from build123d import *

# Parameters (mm, degrees)
F0_R     = 1.5875
F1_DEPTH = 1.524
F2_R     = 1.5875
F3_DEPTH = 4.7752


with BuildPart() as f1:
    # F0 (on Top) → F1 (new body)
    with BuildSketch(Plane.XY):
        with BuildLine():
            Line((-36.890476, -1.143), (-3.175, -2.38125))
            ThreePointArc((-3.175, -2.38125), (3.96875, 0), (-3.175, 2.38125))
            Line((-3.175, 2.38125), (-36.890476, 1.143))
            ThreePointArc((-36.890476, 1.143), (-43.0276, 0), (-36.890476, -1.143))
        make_face()
        with Locations((-39.8526, 0)):
            Circle(F0_R, mode=Mode.SUBTRACT)
        Circle(F0_R, mode=Mode.SUBTRACT)
    extrude(amount=F1_DEPTH)

    # F2 (on face) → F3 (join)
    with BuildSketch(Plane.XY.offset(1.524)):
        with Locations((-39.8526, 0)):
            Circle(F2_R)
        Circle(F2_R)
    extrude(amount=-F3_DEPTH)


solid = f1.part
Part model, mm, in its own coordinate system. A direction names the side the tool comes from. Coordinates: 2 decimals unless noted, no trailing zeros. Write each loop counter-clockwise with the first axis right and the second up, starting at its lowest first coordinate (ties: lowest second). Pieces come first, ordered by that corner, then holes. Notation, with made-up numbers: M 69.25,24 L 96.25,24 A16 cw 96.25,53 Z; hole C 75.5,83 d5. An arc over 180 degrees is marked long. Return JSON: item names as keys, results as strings.
1. Flat gauge pins, fed straight in: pin 1 Ø3 at (x, y) = (-20, 2.5) entering from -Z; pin 2 Ø1 at (x, z) = (-28.5, 0) entering from +Y. Where does each tip first touch, or does it go through?
Determined:
{"pin 1": "z = 0", "pin 2": "y = 1.47"}
2. Saw through at C-C, the plane z = -0.5. Write the cut outline in (x, y) (1 decimal).
Determined:
{"outline": "C -39.9,0 d3.2; C 0,0 d3.2"}
3. 3-axis set-ups, long thin cutter, end or side, ignore diameter. For faces 3 (the face through (-20.269, -1.753, 0.751)), 4 (the face through (-0.34, -1.55, -1.6)), 5 (the face through (-40, 0, -3.251)): which of +Z, -Z, +X, -X, +Y, -Y reach the whole face in a straight line?
Determined:
{"face 3": "+Z, -Z, -Y", "face 4": "-Z", "face 5": "-Z, +X, -X, +Y, -Y"}
4. Saw through at B-B, the plane y = 0. Write the cut outline in (x, z).
Determined:
{"outline": "M -43.03,0 L -41.44,0 L -41.44,-3.25 L -38.27,-3.25 L -38.27,0 L -1.59,0 L -1.59,-3.25 L 1.59,-3.25 L 1.59,0 L 3.97,0 L 3.97,1.52 L -43.03,1.52 Z"}
5. Saw through at A-A, the plane x = 0. Write the cut outline in (y, z).
Determined:
{"outline": "M -3.97,0 L -1.59,0 L -1.59,-3.25 L 1.59,-3.25 L 1.59,0 L 3.97,0 L 3.97,1.52 L -3.97,1.52 Z"}
6. Pull direction X, two halves, no side cores. Call faces 1 (the face through (-19.8, 1.77, 0.75)), 2 (the face through (0, 0, -3.251)): pulls with the +X half, pulls with the -X half, needs draft (parallel to the pull), parting line crosses it, or undercut.
Determined:
{"face 1": "undercut", "face 2": "needs draft"}
7. Probe L1, parallel to Z at x = -40.5, y = -1.75; L2, parallel to X at y = 1, z = -2.95; L3, parallel to Y at x = -5.5, z = 0.6. List the from-to ranges inside material, lowest first.
Determined:
{"L1": "0 to 1.52", "L2": "-41.09 to -38.62, -1.23 to 1.23", "L3": "-2.3 to 2.3"}
